from build123d import *

# Parameters (mm, degrees)
SKETCH1_R                = 50
SKETCH1_R_2              = 48
EXTRUDE1_DEPTH           = 9.5
EXTRUDE2_DEPTH           = 2.5
SKETCH3_R                = 1.45
EXTRUDE3_DEPTH           = 2.5
FILLET1_R                = 2
CIRPATTERN1_COUNT        = 3
FILLET1_OF_CIRPATTERN1_R = 2


with BuildPart() as part:
    # Sketch1 → Extrude1 (new body)
    with BuildSketch(Plane.XY):
        Circle(SKETCH1_R)
        Circle(SKETCH1_R_2, mode=Mode.SUBTRACT)
    extrude(amount=EXTRUDE1_DEPTH)

    # Sketch2 → Extrude2 (add)
    with BuildSketch(Plane.XY):
        with BuildLine():
            Line((-4, 47.833042972), (-4, 41.809089921))
            ThreePointArc((-4, 41.809089921), (0, 42), (4, 41.809089921))
            Line((4, 41.809089921), (4, 47.833042972))
            ThreePointArc((4, 47.833042972), (0, 48), (-4, 47.833042972))
        make_face()
    extrude2 = extrude(amount=EXTRUDE2_DEPTH)

    # Sketch3 → Extrude3 (cut)
    with BuildSketch(Plane.XY.offset(2.5)):
        with Locations((0, 44.5)):
            Circle(SKETCH3_R)
    extrude3 = extrude(amount=-EXTRUDE3_DEPTH, mode=Mode.SUBTRACT)

    # Fillet1
    fillet1_edges = [part.edges().sort_by_distance(p)[0] for p in [
        (4, 47.833042972, 1.25),
        (-4, 47.833042972, 1.25),
        (-4, 41.809089921, 1.25),
        (4, 41.809089921, 1.25),
    ]]
    fillet(fillet1_edges, radius=FILLET1_R)

    # CirPattern1: Extrude2, Extrude3 ×3 about axis
    cirpattern1_axis = Axis((0, 0, 0), (0, 0, 1))
    for i in range(1, CIRPATTERN1_COUNT):
        add(extrude2.rotate(cirpattern1_axis, i * 360 / CIRPATTERN1_COUNT))
        add(extrude3.rotate(cirpattern1_axis, i * 360 / CIRPATTERN1_COUNT), mode=Mode.SUBTRACT)

    # Fillet1 of CirPattern1
    fillet1_of_cirpattern1_edges = [part.edges().sort_by_distance(p)[0] for p in [
        (-43.424630354, -20.452419871, 1.25),
        (-39.424630354, -27.380623101, 1.25),
        (-34.20773398, -24.368646576, 1.25),
        (-38.20773398, -17.440443345, 1.25),
        (39.424630354, -27.380623101, 1.25),
        (43.424630354, -20.452419871, 1.25),
        (38.20773398, -17.440443345, 1.25),
        (34.20773398, -24.368646576, 1.25),
    ]]
    fillet(fillet1_of_cirpattern1_edges, radius=FILLET1_OF_CIRPATTERN1_R)


solid = part.part
Geometry check sheet. Reference: the model listing, model coordinates, mm. A direction names the side the tool comes from. Give positions to 0.01 mm unless a question says otherwise; leave off trailing zeros. Loops run counter-clockwise (first coordinate to the right, second up) from the corner with the lowest first, then second, coordinate; pieces in that order, holes last. Notation, with made-up numbers: (37.5, -14.75) -> (60.5, -14.75) arc R36 cw to (60.5, 20.25) -> close; hole circle Ø10 at (23.25, 87.5). An arc over 180 degrees is marked (long way). Answer in a Markdown table with one row per item. Add a question column.
1) Gauge pin test, flat ends, axial feed: P1, Ø2.5, axis at x = 38.54, y = -22.25, coming from the +Z side; P2, Ø3, axis at x = -0.5, y = 46, coming from the +Z side; P3, Ø5, axis at x = 31.5, z = 1.5, coming from the -Y side; P4, Ø0.8, axis at y = 45, z = 1, coming from the +X side. Record the tip position at first contact, or that the pin passes through.
2) Cross-section at B-B on y = 12.5. Record the boundary of the cut face in (x, z).
3) Cross-section at C-C on z = 5.25. Record the boundary of the cut face in (x, y), and give its area (3 significant figures).
4) Material ranges on probe 1 along Y at (x, z) = (1, 7.5); probe 2 along Y at (x, z) = (3.5, 6); probe 3 along Y at (x, z) = (-38, 1.5), recorded low to high. Write a range as from..to.
5) Set-up check for faces 1 (the face through (36.8, -22, 0)), 2 (the face through (-40, -23, 2.5)), 3 (the face through (0, 42, 1)): record each of +Z, -Z, +X, -X, +Y, -Y from which the full face is reachable in a straight line by a thin tool's end or side.
6) Draft check along X on faces 4 (the face through (47.69, 15.02, 4.68)), 5 (the face through (38.53, -18.32, 1.27)), 6 (the face through (-19, 45, 9.5)). Enter one of: pulls with the +X half, pulls with the -X half, needs draft (parallel to the pull), parting line crosses it, or undercut.
7) Cross-section at D-D on x = -21.5. Record the boundary of the cut face in (y, z).
8) Cross-section at A-A on x = 0. Record the boundary of the cut face in (y, z).
Outcome:
| question | item | result |
|---|---|---|
| 1 | P1 | passes through |
| 1 | P2 | stops at z = 2.5 |
| 1 | P3 | stops at y = -40.73 |
| 1 | P4 | stops at x = 22.6 |
| 2 | outline | (-48.41, 0) -> (-46.34, 0) -> (-46.34, 9.5) -> (-48.41, 9.5) -> close; (46.34, 0) -> (48.41, 0) -> (48.41, 9.5) -> (46.34, 9.5) -> close |
| 3 | outline | circle Ø100 at (0, 0); hole circle Ø96 at (0, 0) |
| 3 | area | 616 mm^2 |
| 4 | probe 1 | y = -49.99..-47.99, 47.99..49.99 |
| 4 | probe 2 | y = -49.88..-47.87, 47.87..49.88 |
| 4 | probe 3 | y = -32.5..-29.33, -26.68..-23.6, -20.9..-18.55, 29.33..32.5 |
| 5 | face 1 | -Z, +X, -X, +Y, -Y |
| 5 | face 2 | +Z |
| 5 | face 3 | +Z, -Z |
| 6 | face 4 | parting line crosses it |
| 6 | face 5 | undercut |
| 6 | face 6 | needs draft |
| 7 | outline | (-45.14, 0) -> (-42.92, 0) -> (-42.92, 9.5) -> (-45.14, 9.5) -> close; (42.92, 0) -> (45.14, 0) -> (45.14, 9.5) -> (42.92, 9.5) -> close |
| 8 | outline | (-50, 0) -> (-48, 0) -> (-48, 9.5) -> (-50, 9.5) -> close; (42, 0) -> (43.05, 0) -> (43.05, 2.5) -> (42, 2.5) -> close; (45.95, 0) -> (50, 0) -> (50, 9.5) -> (48, 9.5) -> (48, 2.5) -> (45.95, 2.5) -> close |
